Can you work these out from the model? Positions are in its coordinate system, mm. Give positions to 0.01 mm unless a question says otherwise; leave off trailing zeros. Order: outer loops, then holes, each group sorted by start corner. A loop starts at its lowest first (then second) coordinate and runs counter-clockwise, first axis right, second up. Notation, with made-up numbers: (-32, 15.5) - (3, 15.5) arc R23 cw to (3, 27.5) - close; hole circle Ø6 at (23, 57.5). An arc over 180 degrees is marked (long way). Answer as CSV lines item,"result".
```python
from build123d import *

# Parameters (mm, degrees)
F0_W     = 23
F0_H     = 25
F0_R     = 8.5
F1_DEPTH = 20
F3_D     = 3.3


with BuildPart() as f1:
    # F0 (on Top) → F1 (new body)
    with BuildSketch(Plane.XY):
        with Locations((-24.353659, 12.5)):
            Rectangle(F0_W, F0_H)
        with Locations((-24.353659, 12.5)):
            Circle(F0_R, mode=Mode.SUBTRACT)
    extrude(amount=F1_DEPTH)

    # F3 (through all)
    with Locations(Plane(origin=(-35.853659, 0, 0), x_dir=(0, -1, 0), z_dir=(-1, 0, 0))):
        with Locations((-2.461657, 2.704677), (-22.262799, 17.144853), (-22.262799, 17.144853)):
            Hole(F3_D / 2)


solid = f1.part
```
1) I want a section at D-D on y = 9.5. Write out the boundary of the cut face in (x, z), plus the area to 3 significant figures.
Answer block:
outline,"(-35.85, 0) - (-32.31, 0) - (-32.31, 20) - (-35.85, 20) - close; (-16.4, 0) - (-12.85, 0) - (-12.85, 20) - (-16.4, 20) - close"
area,"142 mm2"
2) I want a section at C-C on z = 13.75. Write out the boundary of the cut face in (x, y), plus the area to 3 significant figures.
Answer block:
outline,"(-35.85, 0) - (-12.85, 0) - (-12.85, 25) - (-35.85, 25) - close; hole circle Ø17 at (-24.35, 12.5)"
area,"348 mm2"
3) I want a section at A-A on y = 12.5. Write out the boundary of the cut face in (x, z), plus the area to 3 significant figures.
Answer block:
outline,"(-35.85, 0) - (-32.85, 0) - (-32.85, 20) - (-35.85, 20) - close; (-15.85, 0) - (-12.85, 0) - (-12.85, 20) - (-15.85, 20) - close"
area,"120 mm2"
4) If we mould it in two halves opening along Y, with no side actions, what happens to faces 1 (the flat face through (-25, 0, 10)), 2 (the cylindrical face through (-24.193, 23.837, 17.64)), 3 (the flat face through (-35.854, 12, 10))? For each: +Y half, -Y half, draft (parallel to the pull), parting line (faces both ways), or undercut.
Answer block:
face 1,"-Y half"
face 2,"undercut"
face 3,"draft"
5) I'm going to push a flat-ended pin straight in: P1, Ø2, axis at y = 2.46, z = 2.7, coming from the +X side. Where does the tip first touch, or does it pass through?
Answer block:
P1,"through"
6) I need wall thicknesses on line 1 along Z through (x, y) = (-17, 2.5); line 2 along Z through (x, y) = (-30.5, 22.25); line 3 along Y through (x, z) = (-27.75, 16). Which ranges of each line are inside material? Lowest first, please. Write a range as [from, to].
Answer block:
line 1,"[0, 1.06], [4.35, 20]"
line 2,"[0, 15.49], [18.79, 20]"
line 3,"[0, 4.71], [20.29, 21.07], [23.45, 25]"
7) I want a section at B-B on x = -19. Write out the boundary of the cut face in (y, z).
Answer block:
outline,"(0, 0) - (5.9, 0) - (5.9, 20) - (0, 20) - close; (19.1, 0) - (25, 0) - (25, 20) - (19.1, 20) - close; hole circle Ø3.3 at (2.46, 2.7); hole circle Ø3.3 at (22.26, 17.14)"
